Here's the drawing with two shaded views (mm, measured from the low corner). I have some questions. Coordinates: 2 decimals unless noted, no trailing zeros. Write each loop counter-clockwise with the first axis right and the second up, starting at its lowest first coordinate (ties: lowest second). Pieces come first, ordered by that corner, then holes.
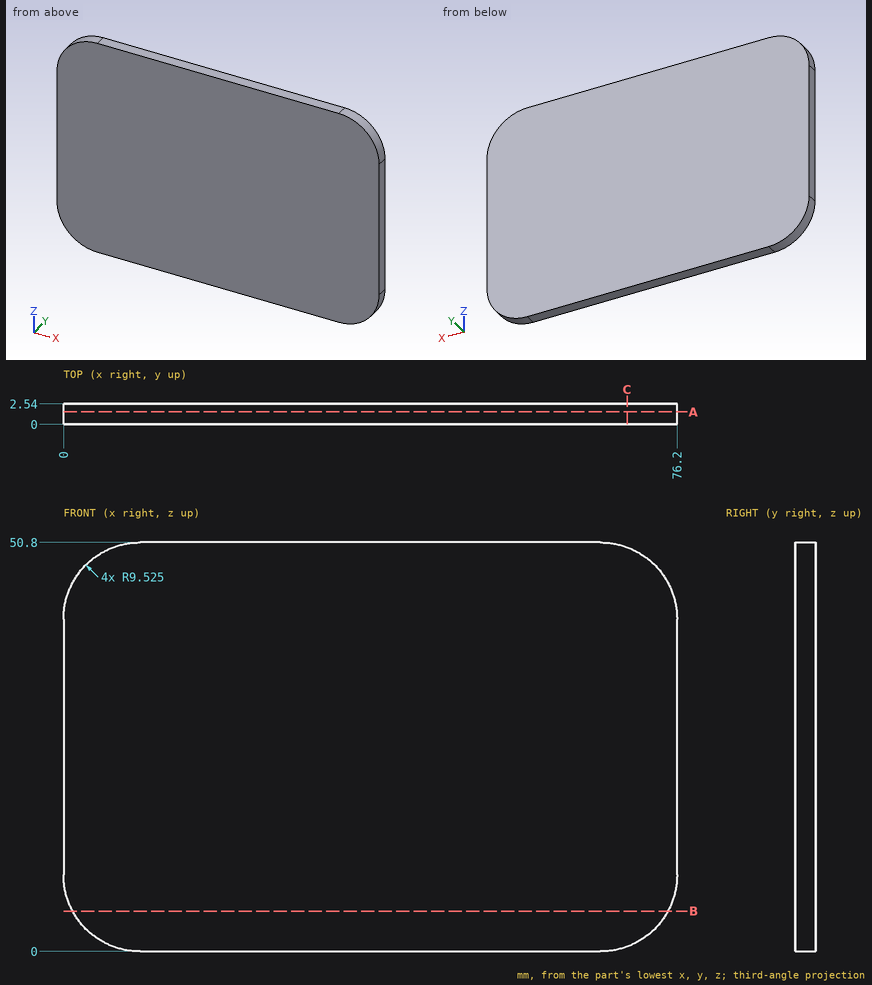
1. Please list where these lines run through material, in increasing order: line 1 along X through (y, z) = (1.7, 9); line 2 along Z through (x, y) = (67, 1.1); line 3 along X through (y, z) = (1.8, 5).
Verdict:
line 1: x = 0.01 to 76.19
line 2: z = 0.01 to 50.79
line 3: x = 1.14 to 75.06
2. I want a section at B-B on z = 5. Please give me the cut outline in (x, y), plus the area to 3 significant figures.
Verdict:
outline: (1.14, 0) - (75.06, 0) - (75.06, 2.54) - (1.14, 2.54) - close
area: 188 mm2
3. I want a section at A-A on y = 1.55. Please give me the cut outline in (x, z) (3 decimals), plus the area to 3 significant figures.
Verdict:
outline: (0, 9.525) arc R9.525 ccw to (9.525, 0) - (66.675, 0) arc R9.525 ccw to (76.2, 9.525) - (76.2, 41.275) arc R9.525 ccw to (66.675, 50.8) - (9.525, 50.8) arc R9.525 ccw to (0, 41.275) - close
area: 3,790 mm2
4. I want a section at C-C on x = 70. Please give me the cut outline in (y, z), plus the area to 3 significant figures.
Verdict:
outline: (0, 0.6) - (2.54, 0.6) - (2.54, 50.2) - (0, 50.2) - close
area: 126 mm2
